Here's how the part is built. I have some questions about the finished solid (model axes, mm). A direction names the side the tool comes from. Give positions to 0.01 mm unless a question says otherwise; leave off trailing zeros. Loops run counter-clockwise (first coordinate to the right, second up) from the corner with the lowest first, then second, coordinate; pieces in that order, holes last. Notation, with made-up numbers: M -25.5,59 L -20.5,59 A11 ccw -20.5,63 Z; hole C 79,-25.5 d8. An arc over 180 degrees is marked long. Write item = value, one per line. Start each with the question number.
```python
from build123d import *

# Parameters (mm, degrees)
SKETCH1_W           = 160
SKETCH1_H           = 200
BOSS_EXTRUDE1_DEPTH = 40
SKETCH2_W           = 20
SKETCH2_H           = 29
CUT_EXTRUDE1_DEPTH  = 42
SKETCH3_R           = 15
CUT_EXTRUDE2_DEPTH  = 25


with BuildPart() as part:
    # Sketch1 → Boss-Extrude1 (new body)
    with BuildSketch(Plane.XY):
        with Locations((0, -20)):
            Rectangle(SKETCH1_W, SKETCH1_H)
    extrude(amount=BOSS_EXTRUDE1_DEPTH)

    # Sketch2 → Cut-Extrude1 (cut)
    with BuildSketch(Plane.XZ.offset(120)):
        with Locations((0, 25.5)):
            Rectangle(SKETCH2_W, SKETCH2_H)
    extrude(amount=-CUT_EXTRUDE1_DEPTH, mode=Mode.SUBTRACT)

    # Sketch3 → Cut-Extrude2 (cut)
    with BuildSketch(Plane.XY.offset(40)):
        with Locations((0, -8)):
            Circle(SKETCH3_R)
    extrude(amount=-CUT_EXTRUDE2_DEPTH, mode=Mode.SUBTRACT)


solid = part.part
```
Q1. If we section it at A-A, the plane z = 18: List the corners of the cut face in (x, y) for me.
Q2. On a 3-axis mill with a long thin cutter (end or side, diameter ignored), from which of +Z, -Z, +X, -X, +Y, -Y can I reach the whole of each face in a straight line? I mean faces 4 (the flat face through (0, -8, 15)), 5 (the flat face through (0, -78, 26)), 6 (the flat face through (-1, -19, 0)). Say none if no direction works.
Q3. If we section it at B-B, the plane y = -8: List the corners of the cut face in (x, z) for me, then the cut area to 3 significant figures.
Q4. Will this pin go through, and if not, where does the flat tip stop? pin 1 (9 mm diameter, centred on x = 7, y = -8, fed in from +Z).
Q5. We'd pull the mould along X, two halves only. Please class faces 1 (the flat face through (-1, 80, 20)), 2 (the flat face through (10, -99, 25)), 3 (the flat face through (-80, -21, 20)): pulls with the +X half, pulls with the -X half, needs draft (parallel to the pull), parting line crosses it, or undercut.
Q6. If we section it at C-C, the plane x = 0: List the corners of the cut face in (y, z) for me.
Q7. If I drill on line 1 along X through (y, z) = (-87, 30.5); line 2 along Y through (x, z) = (0, 27.25); line 3 along X through (y, z) = (-3.5, 27), over which ranges is the centre line in solid material (lowest first)?
Resolved:
q1.outline = M -80,-120 L -10,-120 L -10,-78 L 10,-78 L 10,-120 L 80,-120 L 80,80 L -80,80 Z; hole C 0,-8 d30
q2.face_4 = +Z
q2.face_5 = +Z, -Y
q2.face_6 = -Z, +X, -X, +Y, -Y
q3.outline = M -80,0 L 80,0 L 80,40 L 15,40 L 15,15 L -15,15 L -15,40 L -80,40 Z
q3.area = 5,650 mm²
q4.pin_1 = 15
q5.face_1 = needs draft
q5.face_2 = undercut
q5.face_3 = pulls with the -X half
q6.outline = M -120,0 L 80,0 L 80,40 L 7,40 L 7,15 L -23,15 L -23,40 L -78,40 L -78,11 L -120,11 Z
q7.line_1 = -80 to -10, 10 to 80
q7.line_2 = -78 to -23, 7 to 80
q7.line_3 = -80 to -14.31, 14.31 to 80
